For this review, take the finished solid that the model builds, in its own axes (mm). A direction names the side the tool comes from. Round coordinates to 2 decimals unless told otherwise and drop trailing zeros. Loops run counter-clockwise (first coordinate to the right, second up) from the corner with the lowest first, then second, coordinate; pieces in that order, holes last.
1. Consider section C-C on x = -0.5. State the section outline as (y, z) points (3 decimals), then the cut area to 3 significant figures.
2. Consider section D-D on z = -2. State the section outline as (x, y) points.
3. To check wall thickness, follow line 1 along X through (y, z) = (4.2, -8.5) (3 decimals); line 2 along Z through (x, y) = (-1.25, 4.25); line 3 along Z through (x, y) = (3, 3.5). State the ranges of each line that lie inside material, in increasing order.
4. Tool access review of faces 4 (the flat face through (0, 4.385, -9)), 5 (the flat face through (-6, 0, 2)), 6 (the cylindrical face through (0.07, -2.35, -6.49)), 7 (the cylindrical face through (5.05, -0.06, 1.44)), 8 (the flat face through (-6, 0, -8)): name each direction out of +Z, -Z, +X, -X, +Y, -Y from which nothing blocks a thin tool from reaching the whole face with its end or side.
5. Consider section B-B on z = -7.25. State the section outline as (x, y) points (3 decimals), then the cut area to 3 significant figures.
6. Consider section A-A on y = 3.5. State the section outline as (x, z) points, then the cut area to 3 significant figures.
7. Draft analysis for pull direction X (two halves, no side actions). For faces 1 (the flat face through (6, 0, 2)), 2 (the cylindrical face through (-4.45, -0.08, -2.96)), 3 (the cylindrical face through (2.5, 4.13, 1.76)), state which applies: released by +X, released by -X, zero draft, split by the parting line, or undercut.
8. Clearance check with flat-ended pins moving along their axes: pin 1 Ø4 at (x, y) = (-3, -1.5) entering from -Z; pin 2 Ø2.5 at (x, y) = (-6, 0.5) entering from +Z; pin 3 Ø2.5 at (x, y) = (6.5, 0.5) entering from -Z. State where each tip first meets the part, or that it passes through.
Autodesk Inventor part; units mm, degrees
ref_plane "YZ Plane" through (0, 0, 0) normal (1, 0, 0) x (0, 1, 0)
ref_plane "XZ Plane" through (0, 0, 0) normal (0, 1, 0) x (-1, 0, 0)
ref_plane "Work Plane1" through (0, 0, -3) normal (0, 0, 1) x (1, 0, 0)
sketch "Sketch1" plane through (0, 0, 0) normal (0, 0, 1) x (1, 0, 0)
  circle A0 centre (-6.35, 0) radius 3.885
  circle A1 centre (6.35, 0) radius 3.885
  arc A2 (4.5733, -3.4549) -> (-4.5733, -3.4549) centre (0, -12.3479) ccw
  line L0 (-6.35, 3.885) -> (6.35, 3.885)
  point P0 (0, 0)
  dimension "d0" = 7.77
  dimension "d1" = 6.35
  dimension "d2" = 7.77
  dimension "d3" = 6.35
  dimension "d5" = 0
  dimension "d6" = 0
  dimension "d7" = 20
extrude "Extrusion1" add sketch "Sketch1" along normal blind 1
sketch "Sketch2" plane through (0, 0, 0) normal (0, 0, -1) x (-1, 0, 0)
  arc A0 (-6.35, 3.885) -> (-4.5733, -3.4549) centre (-6.35, 0) ccw
  arc A1 (4.5733, -3.4549) -> (6.35, 3.885) centre (6.35, 0) ccw
  circle A2 centre (-6.35, 0) radius 1.9
  circle A3 centre (6.35, 0) radius 1.9
  point P0 (4.5733, 3.4549)
  point P1 (-4.5733, 3.4549)
  point P2 (0, 0)
  dimension "d10" = 3.8
  dimension "d11" = 3.8
extrude "Extrusion2" add sketch "Sketch2" along normal blind 6
sketch "Sketch3" plane through (-6.35, 0, -6) normal (0, 0, -1) x (-1, 0, 0)
  circle A0 centre (-12.7, 0) radius 1.9
  circle A1 centre (0, 0) radius 1.9
  arc A2 (-12.7, 3.885) -> (-10.9233, -3.4549) centre (-12.7, 0) ccw
  arc A3 (-1.7767, -3.4549) -> (-10.9233, -3.4549) centre (-6.35, -12.3479) ccw
  arc A4 (-1.7767, -3.4549) -> (0, 3.885) centre (0, 0) ccw
  line L0 (-12.7, 3.885) -> (0, 3.885)
  point P0 (-6.35, 0)
extrude "Extrusion3" add sketch "Sketch3" along normal blind 1 contours A0 | A1 | L0 A4 A3 A2
sketch "Sketch4" plane through (0, 0, 1) normal (0, 0, 1) x (1, 0, 0)
  arc A0 (-6.35, 3.885) -> (-4.5733, -3.4549) centre (-6.35, 0) ccw
  arc A1 (4.5733, -3.4549) -> (6.35, 3.885) centre (6.35, 0) ccw
  circle A2 centre (-6.35, 0) radius 1.3
  circle A3 centre (6.35, 0) radius 1.3
  point P0 (4.5733, 3.4549)
  point P1 (-4.5733, 3.4549)
  point P2 (0, 0)
  dimension "d16" = 2.6
  dimension "d17" = 2.6
extrude "Extrusion4" add sketch "Sketch4" along normal blind 1
sketch "Sketch5" plane through (-6.35, 0, -7) normal (0, 0, -1) x (-1, 0, 0)
  arc A0 (-12.7, 3.885) -> (-10.9233, -3.4549) centre (-12.7, 0) ccw
  arc A1 (-1.7767, -3.4549) -> (0, 3.885) centre (0, 0) ccw
  circle A2 centre (-12.7, 0) radius 1.3
  circle A3 centre (0, 0) radius 1.3
  point P0 (-1.7767, 3.4549)
  point P1 (-10.9233, 3.4549)
  point P2 (-6.35, 0)
  dimension "d20" = 2.6
  dimension "d21" = 2.6
extrude "Extrusion5" add sketch "Sketch5" along normal blind 1
chamfer "Chamfer1" distance 0.1 angle 45 2 edges at (7.65, 0, -8) (-5.05, 0, -8)
chamfer "Chamfer2" distance 0.1 angle 45 2 edges at (5.05, 0, 2) (-7.65, 0, 2)
ref_plane "Work Plane1" through (0, 0, -3) normal (0, 0, 1) x (1, 0, 0)
sketch "Skizze6" plane through (-6.35, 3.885, -6) normal (0, 1, 0) x (1, 0, 0)
  point P0 (6.35, -6)
sketch "Skizze7" plane through (-6.35, 3.885, 0) normal (0, 1, 0) x (1, 0, 0)
  line L0 (12.7, 0) -> (0, 0)
  line L1 (0, 0) -> (0, -5)
  line L2 (0, -5) -> (12.7, -5)
  line L3 (12.7, -5) -> (12.7, 0)
  line L4 (1.9, 6) -> (-1.9, 6)
  line L5 (0, 6) -> (12.7, 6)
  line L6 (12.7, 6) -> (12.7, 11)
  line L7 (12.7, 11) -> (0, 11)
  line L8 (0, 11) -> (0, 6)
  point P0 (6.35, 0)
  dimension "d31" = 5
  dimension "d33" = 5
extrude "Extrusion6" add sketch "Skizze7" along normal blind 0.5
sketch "Skizze8" plane through (-6.35, 4.385, 0) normal (0, 1, 0) x (1, 0, 0)
  line L0 (6.35, 0) -> (6.35, -2.5)
  line L1 (6.35, -2.5) -> (3.175, -2.5)
  line L2 (6.35, -2.5) -> (9.525, -2.5)
  line L3 (10.9233, 6) -> (1.7767, 6)
  line L4 (6.35, 6) -> (6.35, 8.5)
  line L5 (6.35, 8.5) -> (3.175, 8.5)
  line L6 (6.35, 8.5) -> (9.525, 8.5)
  dimension "d36" = 2.5
  dimension "d37" = 3.175
  dimension "d38" = 3.175
  dimension "d39" = 2.5
  dimension "d40" = 3.175
  dimension "d41" = 3.175
hole "Bohrung1" at (-3.175, 4.385, 2.5) at (3.175, 4.385, 2.5) at (-3.175, 4.385, -8.5) at (3.175, 4.385, -8.5) direction (0, -1, 0) diameter 2 end through all
equation "\"d2\" = d0"
equation "\"d7\" = d4"
equation "\"d11\" = d10"
equation "\"d17\" = d16"
equation "\"d20\" = d16"
equation "\"d21\" = d16"
properties part number "ConnectingLinks"
Resolved:
1. outline: (-2.36, -7) - (3.885, -7) - (3.885, -11) - (4.385, -11) - (4.385, -6) - (-2.36, -6) - close; (-2.36, 0) - (4.385, 0) - (4.385, 5) - (3.885, 5) - (3.885, 1) - (-2.36, 1) - close
1. area: 17.5 mm2
2. outline: circle Ø3.8 at (-6.35, 0); circle Ø3.8 at (6.35, 0)
3. line 1: x = -6.35 to -4.175, -2.175 to 2.175, 4.175 to 6.35
3. line 2: z = -11 to -6, 0 to 5
3. line 3: z = -7 to -6, 0 to 1
4. face 4: +Z, -Z, +X, -X, +Y
4. face 5: +Z, +X, -X, -Y
4. face 6: +Z, -Z, -Y
4. face 7: +Z
4. face 8: -Z, +X, -X, -Y
5. outline: circle Ø2.6 at (-6.35, 0); (-6.35, 3.885) - (6.35, 3.885) - (6.35, 4.385) - (-6.35, 4.385) - close; circle Ø2.6 at (6.35, 0)
5. area: 17.0 mm2
6. outline: (-8.04, -7) - (8.04, -7) - (8.04, -6) - (-8.04, -6) - close; (-8.04, 0) - (8.04, 0) - (8.04, 1) - (-8.04, 1) - close
6. area: 32.1 mm2
7. face 1: zero draft
7. face 2: undercut
7. face 3: undercut
8. pin 1: stops at z = -7
8. pin 2: stops at z = 2
8. pin 3: stops at z = -8
